Geometry check sheet. Reference: the model listing, model coordinates, mm. Round coordinates to 2 decimals unless told otherwise and drop trailing zeros. Order: outer loops, then holes, each group sorted by start corner. A loop starts at its lowest first (then second) coordinate and runs counter-clockwise, first axis right, second up. Notation, with made-up numbers: (16.25, -2.75) - (24.25, -2.75) arc R20 cw to (24.25, 5.25) - close; hole circle Ø6 at (74, -31.5). An arc over 180 degrees is marked (long way). Use a Markdown table: item, result. Add a question column.
(1) Gauge pin test, flat ends, axial feed: P1, Ø3, axis at y = 5.5, z = 173.5, coming from the +X side; P2, Ø9, axis at x = -1815.77, z = 277.5, coming from the -Y side; P3, Ø6, axis at y = 5, z = 232.5, coming from the +X side; P4, Ø5, axis at y = 7.5, z = 205, coming from the +X side. Record the tip position at first contact, or that the pin passes through.
(2) Thickness scan on line 1 along Z through (x, y) = (-1782, 3.75); line 2 along Z through (x, y) = (-1804.5, 4.75); line 3 along X through (y, z) = (4, 177.5). Record the ranges inside material, lowest first. Write a range as [from, to].
(3) Section check C-C on y = 5. Give the number of separate pieces and of enclosed holes in the cut face, then the cut area to 3 significant figures.
(4) Section check A-A on x = -1871.5. Record the boundary of the cut face in (y, z).
(5) Section check B-B on z = 194.5. Record the boundary of the cut face in (x, y), then the cut area to 3 significant figures.
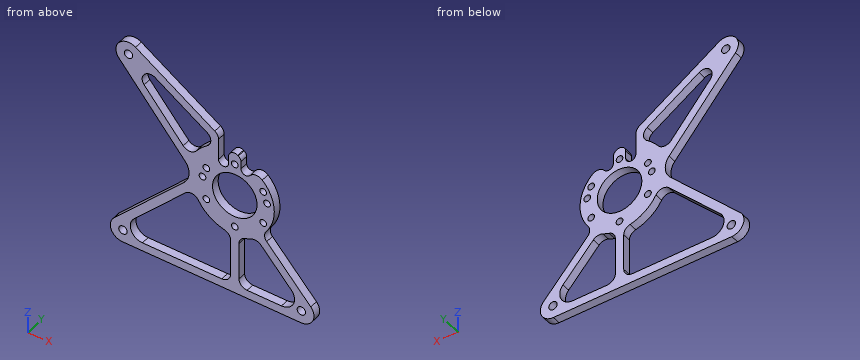
```python
from build123d import *

# Parameters (mm, degrees)
SZKIC3_R                    = 26.5
DODANIE_WYCI_GNI_CIE1_DEPTH = 10
OTW_R1_D                    = 8
OTW_R1_DEPTH                = 10.001
SZYK_KO_OWY1_COUNT          = 18
OTW_R2_D                    = 10
OTW_R2_DEPTH                = 100
OTW_R3_D                    = 10
OTW_R3_DEPTH                = 100
OTW_R4_D                    = 10
OTW_R4_DEPTH                = 10
WYTNIJ_WYCI_GNI_CIE1_DEPTH  = 11
ZAOKR_GLENIE1_R             = 10
OTW_R5_D                    = 10
OTW_R5_DEPTH                = 10
WYTNIJ_WYCI_GNI_CIE2_DEPTH  = 10
ZAOKR_GLENIE2_R             = 10
ZAOKR_GLENIE7_R             = 7


with BuildPart() as part:
    # Szkic3 → Dodanie-wyciągnięcie1 (new body)
    with BuildSketch(Plane(origin=(0, 0, 0), x_dir=(1, 0, 0), z_dir=(0, 1, 0))):
        with BuildLine():
            Line((-1915.5488692, -140.99080739), (-1703.3488692, -133.220934409))
            ThreePointArc((-1703.3488692, -133.220934409), (-1689.223566168, -141.832766807), (-1691.612507096, -158.202886057))
            Line((-1691.612507096, -158.202886057), (-1750, -223.576171044))
            ThreePointArc((-1750, -223.576171044), (-1736.180289372, -268.466810303), (-1768.121254646, -302.904124837))
            Line((-1768.121254646, -302.904124837), (-1899.97553639, -391.673040436))
            ThreePointArc((-1899.97553639, -391.673040436), (-1919.48315677, -389.285445814), (-1919.883316335, -369.636330483))
            Line((-1919.883316335, -369.636330483), (-1840.970754815, -274.791431046))
            ThreePointArc((-1840.970754815, -274.791431046), (-1836.372380588, -260.955992635), (-1842.387744834, -247.675187141))
            Line((-1842.387744834, -247.675187141), (-1925.46803839, -166.72414018))
            ThreePointArc((-1925.46803839, -166.72414018), (-1928.996219751, -150.585779938), (-1915.5488692, -140.99080739))
        make_face()
        with Locations((-1782, -258)):
            Circle(SZKIC3_R, mode=Mode.SUBTRACT)
    extrude(amount=DODANIE_WYCI_GNI_CIE1_DEPTH)

    # Otwór1
    with Locations(Plane(origin=(0, 0, 0), x_dir=(-1, 0, 0), z_dir=(0, -1, 0))):
        with Locations((1782, -219)):
            otw_r1 = Hole(OTW_R1_D / 2, depth=OTW_R1_DEPTH)

    # Szyk kołowy1: Otwór1 ×18 about axis, 10 skipped
    szyk_ko_owy1_axis = Axis((-1782, 10, 258), (0, -1, 0))
    add([otw_r1.rotate(szyk_ko_owy1_axis, i * 360 / SZYK_KO_OWY1_COUNT) for i in range(1, SZYK_KO_OWY1_COUNT) if i not in (1, 2, 4, 7, 8, 10, 11, 14, 16, 17)], mode=Mode.SUBTRACT)

    # Otwór2
    with Locations(Plane(origin=(0, 0, 0), x_dir=(-1, 0, 0), z_dir=(0, -1, 0))):
        with Locations((1702.8, -148.210889132)):
            Hole(OTW_R2_D / 2, depth=OTW_R2_DEPTH)

    # Otwór3
    with Locations(Plane(origin=(0, 0, 0), x_dir=(-1, 0, 0), z_dir=(0, -1, 0))):
        with Locations((1915, -155.980762114)):
            Hole(OTW_R3_D / 2, depth=OTW_R3_DEPTH)

    # Otwór4
    with Locations(Plane(origin=(0, 0, 0), x_dir=(-1, 0, 0), z_dir=(0, -1, 0))):
        with Locations((1908.352535431, -379.230135346)):
            Hole(OTW_R4_D / 2, depth=OTW_R4_DEPTH)

    # Szkic14 → Wytnij-wyciągnięcie1 (cut, through all)
    with BuildSketch(Plane(origin=(0, 0, 0), x_dir=(-1, 0, 0), z_dir=(0, -1, 0))):
        with BuildLine():
            Line((1830.387794708, -245.405504247), (1901.759731773, -175.862742881))
            ThreePointArc((1901.759731773, -175.862742881), (1905.287913135, -159.724382638), (1891.840562583, -150.129410091))
            Line((1891.840562583, -150.129410091), (1787, -146.290588911))
            Line((1787, -146.290588911), (1787, -208.250628145))
            ThreePointArc((1787, -208.250628145), (1814.522074972, -220.02218227), (1830.387794708, -245.405504247))
        make_face()
        with BuildLine():
            Line((1777, -208.250628145), (1777, -145.9244309))
            Line((1777, -145.9244309), (1726.449545971, -144.073485533))
            ThreePointArc((1726.449545971, -144.073485533), (1712.324242939, -152.685317931), (1714.713183868, -169.05543718))
            Line((1714.713183868, -169.05543718), (1756.005588073, -215.288285581))
            ThreePointArc((1756.005588073, -215.288285581), (1766.10831827, -210.592675125), (1777, -208.250628145))
        make_face()
        with BuildLine():
            Line((1889.850904158, -349.175505229), (1834.500977493, -282.650504301))
            ThreePointArc((1834.500977493, -282.650504301), (1820.727394871, -301.176253734), (1800.818732436, -312.86214824))
            Line((1800.818732436, -312.86214824), (1876.579050862, -363.866645198))
            ThreePointArc((1876.579050862, -363.866645198), (1889.584131115, -362.27491545), (1889.850904158, -349.175505229))
        make_face()
    extrude(amount=-WYTNIJ_WYCI_GNI_CIE1_DEPTH, mode=Mode.SUBTRACT)

    # Zaokrąglenie1
    zaokr_glenie1_edges = [part.edges().sort_by_distance(p)[0] for p in [
        (-1800.818732436, 5, 312.86214824),
        (-1834.500977493, 5, 282.650504301),
        (-1777, 5, 208.250628145),
        (-1756.005588073, 5, 215.288285581),
        (-1777, 5, 145.9244309),
        (-1830.387794708, 5, 245.405504247),
        (-1787, 5, 208.250628145),
        (-1787, 5, 146.290588911),
        (-1750, 5, 223.576171044),
        (-1768.121254646, 5, 302.904124837),
    ]]
    fillet(zaokr_glenie1_edges, radius=ZAOKR_GLENIE1_R)

    # Otwór5
    with Locations(Plane(origin=(0, 0, 0), x_dir=(-1, 0, 0), z_dir=(0, -1, 0))):
        with Locations((1795.33878559, -294.648012211), (1768.66121441, -294.648012211)):
            Hole(OTW_R5_D / 2, depth=OTW_R5_DEPTH)

    # Szkic18 → Wytnij-wyciągnięcie2 (cut)
    with BuildSketch(Plane(origin=(0, 0, 0), x_dir=(-1, 0, 0), z_dir=(0, -1, 0))):
        with BuildLine():
            Line((1762.66121441, -294.648012211), (1762.66121441, -300.837032716))
            ThreePointArc((1762.66121441, -300.837032716), (1764.765334946, -301.7260371), (1766.910163713, -302.511760703))
            ThreePointArc((1766.910163713, -302.511760703), (1768.13628585, -303.020458445), (1769.284226275, -303.687078026))
            Line((1769.284226275, -303.687078026), (1774.66121441, -307.307054561))
            Line((1774.66121441, -307.307054561), (1774.66121441, -294.648012211))
            ThreePointArc((1774.66121441, -294.648012211), (1768.66121441, -288.648012211), (1762.66121441, -294.648012211))
        make_face()
        with BuildLine():
            Line((1789.33878559, -294.648012211), (1789.33878559, -317.188508997))
            Line((1789.33878559, -317.188508997), (1801.33878559, -325.267328836))
            Line((1801.33878559, -325.267328836), (1801.33878559, -294.648012211))
            ThreePointArc((1801.33878559, -294.648012211), (1795.33878559, -288.648012211), (1789.33878559, -294.648012211))
        make_face()
    extrude(amount=-WYTNIJ_WYCI_GNI_CIE2_DEPTH, mode=Mode.SUBTRACT)

    # Zaokrąglenie2
    zaokr_glenie2_edges = [part.edges().sort_by_distance(p)[0] for p in [
        (-1762.66121441, 5, 300.837032716),
        (-1801.33878559, 5, 325.267328836),
    ]]
    fillet(zaokr_glenie2_edges, radius=ZAOKR_GLENIE2_R)

    # Zaokrąglenie7
    zaokr_glenie7_edges = [part.edges().sort_by_distance(p)[0] for p in [
        (-1774.66121441, 5, 307.307054561),
        (-1789.33878559, 5, 317.188508997),
    ]]
    fillet(zaokr_glenie7_edges, radius=ZAOKR_GLENIE7_R)


solid = part.part
```
Check sheet entries:
| question | item | result |
|---|---|---|
| 1 | P1 | stops at x = -1703.94 |
| 1 | P2 | stops at y = 0 |
| 1 | P3 | stops at x = -1740.74 |
| 1 | P4 | stops at x = -1731.18 |
| 2 | line 1 | z = [136.1, 215], [223, 231.5], [284.5, 293], [301, 311.03] |
| 2 | line 2 | z = [136.92, 146.93], [213.35, 244], [272, 327.24] |
| 2 | line 3 | x = [-1914.41, -1900.08], [-1787, -1777], [-1722.26, -1708.85] |
| 3 | separate pieces | 1 |
| 3 | enclosed holes | 15 |
| 3 | area | 14,000 mm2 |
| 4 | outline | (0, 139.38) - (10, 139.38) - (10, 149.38) - (0, 149.38) - close; (0, 205.35) - (10, 205.35) - (10, 219.31) - (0, 219.31) - close; (0, 311.48) - (10, 311.48) - (10, 327.12) - (0, 327.12) - close; (0, 360.45) - (10, 360.45) - (10, 372.5) - (0, 372.5) - close |
| 5 | outline | (-1896.96, 0) - (-1882.63, 0) - (-1882.63, 10) - (-1896.96, 10) - close; (-1787, 0) - (-1777, 0) - (-1777, 10) - (-1787, 10) - close; (-1737.44, 0) - (-1724.03, 0) - (-1724.03, 10) - (-1737.44, 10) - close |
| 5 | area | 377 mm2 |
